from build123d import *

# Parameters (mm, degrees)
F0_R     = 3.81
F1_DEPTH = 2.921
F2_R     = 1.4605
F3_R     = 1.9685
F4_DEPTH = 12.319


with BuildPart() as f1:
    # F0 (on Right) → F1 (new body)
    with BuildSketch(Plane.YZ):
        Circle(F0_R)
    extrude(amount=-F1_DEPTH)

    # F2
    f2_edges = [f1.edges().sort_by_distance(p)[0] for p in [
        (0, -3.81, 0),
    ]]
    fillet(f2_edges, radius=F2_R)

    # F3 (on face) → F4 (join)
    with BuildSketch(Plane(origin=(-2.921, 0, 0), x_dir=(0, -1, 0), z_dir=(-1, 0, 0))):
        Circle(F3_R)
    extrude(amount=F4_DEPTH)


solid = f1.part
Part model, mm, in its own coordinate system. A direction names the side the tool comes from. Round coordinates to 2 decimals unless told otherwise and drop trailing zeros. Order: outer loops, then holes, each group sorted by start corner. A loop starts at its lowest first (then second) coordinate and runs counter-clockwise, first axis right, second up. Notation, with made-up numbers: (8, 67) -> (58, 67) arc R28 ccw to (58, 97) -> close; hole circle Ø7 at (27, 61). An arc over 180 degrees is marked (long way). Put each result on its own line as item: value.
Q1. Band-saw the part on D-D (x = -2.75). Give the cut face in (y, z), and give its area (3 significant figures).
From the geometry:
outline: circle Ø7.62 at (0, 0)
area: 45.6 mm2
Q2. Pin check, flat tips, straight feed: pin 1 Ø2 at (x, z) = (-6, -1) entering from -Y; pin 2 Ø2 at (x, y) = (-5, 0) entering from +Z. Stop position of each tip, or through.
From the geometry:
pin 1: stops at y = -1.97
pin 2: stops at z = 1.97
Q3. Wall check: line 1 (X direction, y = -1.25, z = 1.75); line 2 (Y direction, x = -7, z = -0.75); line 3 (X direction, y = 3, z = -1). Give the ranges that are in metal, low to high. Write a range as [from, to].
From the geometry:
line 1: x = [-2.92, 0]
line 2: y = [-1.82, 1.82]
line 3: x = [-2.92, -0.25]
Q4. Band-saw the part on A-A (z = 0). Give the cut face in (x, y), and give its area (3 significant figures).
From the geometry:
outline: (-15.24, -1.97) -> (-2.92, -1.97) -> (-2.92, -3.81) -> (-1.46, -3.81) arc R1.46 ccw to (0, -2.35) -> (0, 2.35) arc R1.46 ccw to (-1.46, 3.81) -> (-2.92, 3.81) -> (-2.92, 1.97) -> (-15.24, 1.97) -> close
area: 69.8 mm2
Q5. Tool access for faces 1 (the face through (-15.24, 0, 0)), 2 (the face through (-2.921, 2, -2)): list every direction of +Z, -Z, +X, -X, +Y, -Y with a clear straight run to the whole face (end or side of a thin tool).
From the geometry:
face 1: +Z, -Z, -X, +Y, -Y
face 2: -X
Q6. Band-saw the part on C-C (x = -5.5). Give the cut face in (y, z), and give its area (3 significant figures).
From the geometry:
outline: circle Ø3.94 at (0, 0)
area: 12.2 mm2
